```python
from build123d import *

# Parameters (mm, degrees)
SKETCH1_W           = 95
SKETCH1_H           = 152.42
BOSS_EXTRUDE1_DEPTH = 5
SKETCH2_R           = 1.75
CUT_EXTRUDE1_DEPTH  = 10
SKETCH3_R           = 3.5
CUT_EXTRUDE2_DEPTH  = 3
CUT_EXTRUDE3_DEPTH  = 10
SKETCH4_R           = 1.75
CUT_EXTRUDE4_DEPTH  = 10
CUT_EXTRUDE5_DEPTH  = 3.5


with BuildPart() as part:
    # Sketch1 → Boss-Extrude1 (new body)
    with BuildSketch(Plane(origin=(0, 0, 0), x_dir=(1, 0, 0), z_dir=(0, 1, 0))):
        Rectangle(SKETCH1_W, SKETCH1_H)
    extrude(amount=BOSS_EXTRUDE1_DEPTH)

    # Sketch2 → Cut-Extrude1 (cut)
    with BuildSketch(Plane.XZ):
        with Locations(Location((42.5, -61.96, 0), (0, 0, 270))):
            Circle(SKETCH2_R)
        with Locations(Location((-42.5, -61.96, 0), (0, 0, 270))):
            Circle(SKETCH2_R)
        with Locations(Location((-42.5, 61.04, 0), (0, 0, 270))):
            Circle(SKETCH2_R)
        with Locations(Location((42.5, 61.04, 0), (0, 0, 270))):
            Circle(SKETCH2_R)
    extrude(amount=-CUT_EXTRUDE1_DEPTH, mode=Mode.SUBTRACT)

    # Sketch3 → Cut-Extrude2 (cut)
    with BuildSketch(Plane.XZ):
        with Locations(Location((42.5, -61.96, 0), (0, 0, 270))):
            Circle(SKETCH3_R)
        with Locations(Location((42.5, 61.04, 0), (0, 0, 270))):
            Circle(SKETCH3_R)
        with Locations(Location((-42.5, 61.04, 0), (0, 0, 270))):
            Circle(SKETCH3_R)
        with Locations(Location((-42.5, -61.96, 0), (0, 0, 270))):
            Circle(SKETCH3_R)
    extrude(amount=-CUT_EXTRUDE2_DEPTH, mode=Mode.SUBTRACT)

    # Sketch5 → Cut-Extrude3 (cut)
    with BuildSketch(Plane.XZ):
        Polygon((39.5, -34.01), (19.5, -34.01), (19.5, -76.21), (-19.5, -76.21), (-19.5, -34.01), (-39.5, -34.01), (-39.5, 9.61), (39.5, 9.61), align=None)
    extrude(amount=-CUT_EXTRUDE3_DEPTH, mode=Mode.SUBTRACT)

    # Sketch4 → Cut-Extrude4 (cut)
    with BuildSketch(Plane.XZ):
        with Locations(Location((28.5, -41.21, 0), (0, 0, 270))):
            Circle(SKETCH4_R)
        with Locations(Location((28.5, 15.79, 0), (0, 0, 270))):
            Circle(SKETCH4_R)
        with Locations(Location((-28.5, 15.79, 0), (0, 0, 270))):
            Circle(SKETCH4_R)
        with Locations(Location((-28.5, -41.21, 0), (0, 0, 270))):
            Circle(SKETCH4_R)
    extrude(amount=-CUT_EXTRUDE4_DEPTH, mode=Mode.SUBTRACT)

    # Sketch6 → Cut-Extrude5 (cut)
    with BuildSketch(Plane(origin=(0, 5, 0), x_dir=(1, 0, 0), z_dir=(0, 1, 0))):
        Polygon((-26.190598923, 45.21), (-30.809401077, 45.21), (-33.118802154, 41.21), (-30.809401077, 37.21), (-26.190598923, 37.21), (-23.881197846, 41.21), align=None)
        Polygon((30.809401077, 45.21), (26.190598923, 45.21), (23.881197846, 41.21), (26.190598923, 37.21), (30.809401077, 37.21), (33.118802154, 41.21), align=None)
        Polygon((30.809401077, -11.79), (26.190598923, -11.79), (23.881197846, -15.79), (26.190598923, -19.79), (30.809401077, -19.79), (33.118802154, -15.79), align=None)
        Polygon((-26.190598923, -19.79), (-23.881197846, -15.79), (-26.190598923, -11.79), (-30.809401077, -11.79), (-33.118802154, -15.79), (-30.809401077, -19.79), align=None)
    extrude(amount=-CUT_EXTRUDE5_DEPTH, mode=Mode.SUBTRACT)


solid = part.part
```
Verification items for the finished model (mm, model axes). A direction names the side the tool comes from. Give positions to 0.01 mm unless a question says otherwise; leave off trailing zeros. Write each loop counter-clockwise with the first axis right and the second up, starting at its lowest first coordinate (ties: lowest second). Pieces come first, ordered by that corner, then holes. Notation, with made-up numbers: (13, 62) - (57, 62) arc R19 ccw to (57, 85) - close; hole circle Ø1 at (34, -23). An arc over 180 degrees is marked (long way). Put each result on its own line as item: value.
Q1. Section check D-D on z = 61.04. Record the cut outline in (x, y).
Result:
outline: (-47.5, 0) - (-46, 0) - (-46, 3) - (-44.25, 3) - (-44.25, 5) - (-47.5, 5) - close; (-40.75, 3) - (-39, 3) - (-39, 0) - (39, 0) - (39, 3) - (40.75, 3) - (40.75, 5) - (-40.75, 5) - close; (44.25, 3) - (46, 3) - (46, 0) - (47.5, 0) - (47.5, 5) - (44.25, 5) - close
Q2. Depth check by flat-ended pin: P1, Ø3.5, axis at x = 41.5, z = 62, coming from the -Y side; P2, Ø2.5, axis at x = -30.5, z = -42, coming from the +Y side; P3, Ø1.5, axis at x = 16.5, y = 2.5, coming from the -Z side; P4, Ø5, axis at x = 21, z = 6, coming from the +Y side. Enter the tip coordinate at first touch or a pass-through.
Result:
P1: y = 3
P2: y = 1.5
P3: z = 9.61
P4: through
Q3. Set-up check for faces 5 (the face through (30, 2, -34.01)), 6 (the face through (-26.5, 1.5, -41.3)), 7 (the face through (19.5, 2, -55)), 8 (the face through (42, 3, -60)): record each of +Z, -Z, +X, -X, +Y, -Y from which the full face is reachable in a straight line by a thin tool's end or side.
Result:
face 5: +Y, -Y
face 6: +Y
face 7: -Z, +Y, -Y
face 8: -Y
Q4. Scan lines: probe 1 along X at (y, z) = (2.25, -61.96); probe 2 along Z at (x, y) = (-43, 0.55); probe 3 along Z at (x, y) = (26.5, 2.1). Record each from-to range of solid material in increasing order. Write a range as from..to.
Result:
probe 1: -47.5..-46, -39..-19.5, 19.5..39, 46..47.5
probe 2: -76.21..-65.42, -58.5..57.58, 64.5..76.21
probe 3: -76.21..-45.21, -37.21..-34.01, 9.61..11.79, 19.79..76.21
Q5. Section check A-A on x = 42.5. Record the cut outline in (y, z), and give its area (3 significant figures).
Result:
outline: (0, -76.21) - (5, -76.21) - (5, -63.71) - (3, -63.71) - (3, -65.46) - (0, -65.46) - close; (0, -58.46) - (3, -58.46) - (3, -60.21) - (5, -60.21) - (5, 59.29) - (3, 59.29) - (3, 57.54) - (0, 57.54) - close; (0, 64.54) - (3, 64.54) - (3, 62.79) - (5, 62.79) - (5, 76.21) - (0, 76.21) - close
area: 706 mm2
Q6. Section check B-B on z = -61.96. Record the cut outline in (x, y).
Result:
outline: (-47.5, 0) - (-46, 0) - (-46, 3) - (-44.25, 3) - (-44.25, 5) - (-47.5, 5) - close; (-40.75, 3) - (-39, 3) - (-39, 0) - (-19.5, 0) - (-19.5, 5) - (-40.75, 5) - close; (19.5, 0) - (39, 0) - (39, 3) - (40.75, 3) - (40.75, 5) - (19.5, 5) - close; (44.25, 3) - (46, 3) - (46, 0) - (47.5, 0) - (47.5, 5) - (44.25, 5) - close
Q7. Mould release check, pull along Z, two halves, no side actions. Record for faces 1 (the face through (33, 2, -76.21)), 2 (the face through (29, 3, -45.21)), 3 (the face through (-19.5, 2, -55)), 4 (the face through (-29, 3, 19.79)): released by +Z, released by -Z, zero draft, split by the parting line, or undercut.
Result:
face 1: released by -Z
face 2: undercut
face 3: zero draft
face 4: undercut
Q8. Section check C-C on x = 28.5. Record the cut outline in (y, z).
Result:
outline: (0, -76.21) - (5, -76.21) - (5, -45.21) - (1.5, -45.21) - (1.5, -42.96) - (0, -42.96) - close; (0, -39.46) - (1.5, -39.46) - (1.5, -37.21) - (5, -37.21) - (5, -34.01) - (0, -34.01) - close; (0, 9.61) - (5, 9.61) - (5, 11.79) - (1.5, 11.79) - (1.5, 14.04) - (0, 14.04) - close; (0, 17.54) - (1.5, 17.54) - (1.5, 19.79) - (5, 19.79) - (5, 76.21) - (0, 76.21) - close
